from build123d import *

# Parameters (mm, degrees)
SKETCH1_W           = 100
SKETCH1_H           = 200
BOSS_EXTRUDE1_DEPTH = 10
SKETCH3_R           = 4
CUT_EXTRUDE2_DEPTH  = 113.249721603
SKETCH4_R           = 4
CUT_EXTRUDE3_DEPTH  = 113.249721603
SKETCH5_R           = 12.5
CUT_EXTRUDE4_DEPTH  = 113.249721603


with BuildPart() as part:
    # Sketch1 → Boss-Extrude1 (new body)
    with BuildSketch(Plane.XY):
        Rectangle(SKETCH1_W, SKETCH1_H)
    extrude(amount=BOSS_EXTRUDE1_DEPTH)

    # Sketch3 → Cut-Extrude2 (cut, through all)
    with BuildSketch(Plane.XY.offset(10)):
        with Locations((0, -75)):
            Circle(SKETCH3_R)
    extrude(amount=-CUT_EXTRUDE2_DEPTH, mode=Mode.SUBTRACT)

    # Sketch4 → Cut-Extrude3 (cut, through all)
    with BuildSketch(Plane.XY.offset(10)):
        with Locations((0, 75)):
            Circle(SKETCH4_R)
    extrude(amount=-CUT_EXTRUDE3_DEPTH, mode=Mode.SUBTRACT)

    # Sketch5 → Cut-Extrude4 (cut, through all)
    with BuildSketch(Plane.XY.offset(10)):
        with Locations((0, 75)):
            Circle(SKETCH5_R)
    extrude(amount=-CUT_EXTRUDE4_DEPTH, mode=Mode.SUBTRACT)


solid = part.part
Could you check a few things on this model? Use its own coordinates, in mm. Give positions to 0.01 mm unless a question says otherwise; leave off trailing zeros. Order: outer loops, then holes, each group sorted by start corner. A loop starts at its lowest first (then second) coordinate and runs counter-clockwise, first axis right, second up. Notation, with made-up numbers: (43, -19) - (101, -19) arc R11 ccw to (101, 0) - close; hole circle Ø9 at (62.25, 30). An arc over 180 degrees is marked (long way). Return JSON: item names as keys, results as strings. Group by question number.
Q1. Please list where these lines run through material, in increasing order: line 1 along Y through (x, z) = (0, 2.75); line 2 along Y through (x, z) = (-1, 5.75); line 3 along X through (y, z) = (72.5, 4.25). Write a range as [from, to].
Q2. Suppose I cut it at D-D, the plane y = -75. Please give me the cut outline in (x, z), and give its area (3 significant figures).
Q3. Will this pin go through, and if not, where does the flat tip stop? pin 1 Ø22.5 at (x, y) = (0, 75) entering from +Z.
Q4. Thinking about a two-plate mould opening in Y: for faces 1 (the face through (-0.867, -78.905, 5.07)), 2 (the face through (-1, 100, 5)), 3 (the face through (-1, -100, 5)), 4 (the face through (-1, 1, 10)), which applies, pulls with the +Y half, pulls with the -Y half, needs draft (parallel to the pull), parting line crosses it, or undercut?
Q5. Suppose I cut it at C-C, the plane z = 3. Please give me the cut outline in (x, y).
Q6. Suppose I cut it at B-B, the plane y = 75. Please give me the cut outline in (x, z), and give its area (3 significant figures).
Q7. Suppose I cut it at A-A, the plane x = 0. Please give me the cut outline in (y, z).
Resolved:
{
 "1": {"line 1": "y = [-100, -79], [-71, 62.5], [87.5, 100]", "line 2": "y = [-100, -78.87], [-71.13, 62.54], [87.46, 100]", "line 3": "x = [-50, -12.25], [12.25, 50]"},
 "2": {"outline": "(-50, 0) - (-4, 0) - (-4, 10) - (-50, 10) - close; (4, 0) - (50, 0) - (50, 10) - (4, 10) - close", "area": "920 mm2"},
 "3": {"pin 1": "passes through"},
 "4": {"face 1": "undercut", "face 2": "pulls with the +Y half", "face 3": "pulls with the -Y half", "face 4": "needs draft"},
 "5": {"outline": "(-50, -100) - (50, -100) - (50, 100) - (-50, 100) - close; hole circle Ø25 at (0, 75); hole circle Ø8 at (0, -75)"},
 "6": {"outline": "(-50, 0) - (-12.5, 0) - (-12.5, 10) - (-50, 10) - close; (12.5, 0) - (50, 0) - (50, 10) - (12.5, 10) - close", "area": "750 mm2"},
 "7": {"outline": "(-100, 0) - (-79, 0) - (-79, 10) - (-100, 10) - close; (-71, 0) - (62.5, 0) - (62.5, 10) - (-71, 10) - close; (87.5, 0) - (100, 0) - (100, 10) - (87.5, 10) - close"}
}
